Verification items for this drawing (mm, ordinates from the low corner). A direction names the side the tool comes from. Round coordinates to 2 decimals unless told otherwise and drop trailing zeros. Order: outer loops, then holes, each group sorted by start corner. A loop starts at its lowest first (then second) coordinate and runs counter-clockwise, first axis right, second up. Notation, with made-up numbers: (6.5, 70) - (56.5, 70) arc R16 cw to (56.5, 80) - close; hole circle Ø2 at (-3, 68.5). An arc over 180 degrees is marked (long way). Return JSON: item names as keys, results as strings. Group by question number.
Q1. Tool access check on the marked faces 1, 2 and 3. Record the directions out of +Z, -Z, +X, -X, +Y, -Y that give a thin tool (end or side, any length) a straight path to the whole face; none if there is none.
Q2. Draft check along Y on the marked faces 4, 5 and 6. Enter one of: pulls with the +Y half, pulls with the -Y half, needs draft (parallel to the pull), parting line crosses it, or undercut.
Q3. Sectioned sample at A-A, the plane z = 1.5. Record the cut outline in (x, y), then the cut area to 3 significant figures.
Q4. Sectioned sample at D-D, the plane x = 39.5. Record the cut outline in (y, z), then the cut area to 3 significant figures.
Q5. Material ranges on line 1 along Y through (x, z) = (68.5, 2.7); line 2 along X through (y, z) = (26, 10); line 3 along X through (y, z) = (18.5, 6.75), recorded low to high.
Q6. Sectioned sample at B-B, the plane y = 17.5. Record the cut outline in (x, z), then the cut area to 3 significant figures.
Q7. Sectioned sample at C-C, the plane z = 9.75. Record the cut outline in (x, y).
Q8. Gauge pin test, flat ends, axial feed: pin 1 Ø9 at (x, z) = (46, 6.5) entering from -Y; pin 2 Ø5 at (y, z) = (15, 6) entering from +X; pin 3 Ø1.5 at (y, z) = (28, 6) entering from -X. Record the tip position at first contact, or that the pin passes through.
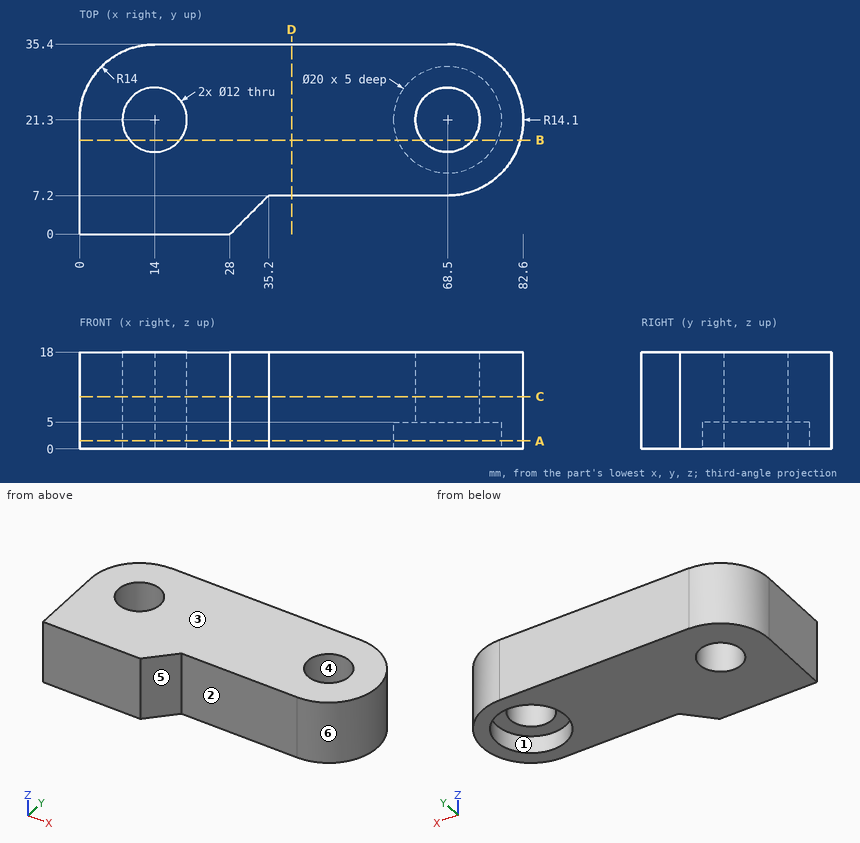
Reply:
{
 "1": {"face 1": "-Z", "face 2": "+Z, -Z, +X, -Y", "face 3": "+Z, +X, -X, +Y, -Y"},
 "2": {"face 4": "undercut", "face 5": "pulls with the -Y half", "face 6": "parting line crosses it"},
 "3": {"outline": "(0, 0) - (28, 0) - (35.2, 7.2) - (68.5, 7.2) arc R14.1 ccw to (68.5, 35.4) - (14, 35.4) - (14, 35.3) arc R14 ccw to (0, 21.3) - close; hole circle Ø12 at (14, 21.3); hole circle Ø20 at (68.5, 21.3)", "area": "2,000 mm^2"},
 "4": {"outline": "(7.2, 0) - (35.4, 0) - (35.4, 18) - (7.2, 18) - close", "area": "508 mm^2"},
 "5": {"line 1": "7.2 to 11.3, 31.3 to 35.4", "line 2": "0.81 to 10.27, 17.73 to 64.77, 72.23 to 81.79", "line 3": "0 to 8.69, 19.31 to 63.19, 73.81 to 82.32"},
 "6": {"outline": "(0, 0) - (9.36, 0) - (9.36, 18) - (0, 18) - close; (18.64, 0) - (59.25, 0) - (59.25, 5) - (63.86, 5) - (63.86, 18) - (18.64, 18) - close; (73.14, 5) - (77.75, 5) - (77.75, 0) - (82.08, 0) - (82.08, 18) - (73.14, 18) - close", "area": "1,100 mm^2"},
 "7": {"outline": "(0, 0) - (28, 0) - (35.2, 7.2) - (68.5, 7.2) arc R14.1 ccw to (68.5, 35.4) - (14, 35.4) - (14, 35.3) arc R14 ccw to (0, 21.3) - close; hole circle Ø12 at (14, 21.3); hole circle Ø12 at (68.5, 21.3)"},
 "8": {"pin 1": "y = 7.2", "pin 2": "x = 82.08", "pin 3": "x = 1.33"}
}
